Work out the finished part from the listing and answer in its coordinate system (mm). A direction names the side the tool comes from. Coordinates: 2 decimals unless noted, no trailing zeros. Write each loop counter-clockwise with the first axis right and the second up, starting at its lowest first coordinate (ties: lowest second). Pieces come first, ordered by that corner, then holes. Notation, with made-up numbers: (70, -26) - (105, -26) arc R18 ccw to (105, -14) - close; hole circle Ø1 at (-40, 61). An arc over 180 degrees is marked (long way). Use a Markdown table: item, result. Add a question column.
(1) For a pull along X with two mould halves and no side action, classify faces 1 (the face through (0.616, 2.014, 1.088)), 2 (the face through (-1.5, 3, 0)), 3 (the face through (-1.5, -7.4, -0.07)) as released by +X, released by -X, zero draft, split by the parting line, or undercut.
(2) The part is cut by section A-A, the plane z = 0. Give the vertices of the cut face in (x, y).
(3) Given pin 1 Ø3 at (x, y) = (-0.5, -13) entering from +Z; pin 2 Ø0.8 at (x, z) = (0, 0) entering from +Y, each flat-ended and moving along its own axis, determine where each tip first touches the part or whether it passes through.
(4) Find the intervals of material crossed by line 1 (Y direction, x = -1.05, z = 0.8); line 2 (Y direction, x = 0.6, z = 1.85); line 3 (Z direction, x = 0, y = -3.25), in increasing order. Write a range as from..to.
(5) The part is cut by section B-B, the plane y = -12.5. Give the vertices of the cut face in (x, z), then the cut area to 3 significant figures.
(6) A tool of negligible diameter and unlimited length cuts with its end or side. For faces 4 (the face through (0, -15, 0)), 5 (the face through (-2, 0, 0)), 6 (the face through (0, 1, 0)), from which of +Z, -Z, +X, -X, +Y, -Y can it reach the whole face along a straight path? Write none if from no direction.
Autodesk Inventor part; units mm, degrees
ref_plane "YZ Plane" through (0, 0, 0) normal (1, 0, 0) x (0, 1, 0)
ref_plane "XZ Plane" through (0, 0, 0) normal (0, 1, 0) x (-1, 0, 0)
ref_plane "XY Plane" through (0, 0, 0) normal (0, 0, 1) x (1, 0, 0)
sketch "スケッチ1" plane through (0, 0, 0) normal (0, 1, 0) x (-1, 0, 0)
  circle A0 centre (0, 0) radius 2.75
  dimension "d0" = 5.5
extrude "押し出し1" add sketch "スケッチ1" along normal blind 3
sketch "スケッチ2" plane through (0, 0, 0) normal (0, -1, 0) x (1, 0, 0)
  circle A0 centre (0, 0) radius 1.5
  dimension "d3" = 3
extrude "押し出し2" add sketch "スケッチ2" along normal blind 15
fillet "フィレット1" radius 0.5 1 edges at (2.75, 3, 0)
fillet "フィレット1" radius 0.2 1 edges at (2.75, 0, 0)
sketch "スケッチ3" plane through (0, 3, 0) normal (0, 1, 0) x (1, 0, 0)
  line L0 (0, 1.4434) -> (-1.25, 0.7217)
  line L1 (-1.25, 0.7217) -> (-1.25, -0.7217)
  line L2 (-1.25, -0.7217) -> (0, -1.4434)
  line L3 (0, -1.4434) -> (1.25, -0.7217)
  line L4 (1.25, -0.7217) -> (1.25, 0.7217)
  line L5 (1.25, 0.7217) -> (0, 1.4434)
  line L6 (0, 1.4434) -> (0, -1.4434) construction
  circle A0 centre (0, 0) radius 1.4434 construction
  dimension "d12" = 2.5
extrude "押し出し3" cut sketch "スケッチ3" against normal blind 2
thread "ねじ1"
properties part number "M3-CapScrew"
Model answer:
| question | item | result |
|---|---|---|
| 1 | face 1 | undercut |
| 1 | face 2 | zero draft |
| 1 | face 3 | split by the parting line |
| 2 | outline | (-2.75, 0.2) arc R0.2 ccw to (-2.55, 0) - (-1.5, 0) - (-1.5, -15) - (1.5, -15) - (1.5, 0) - (2.55, 0) arc R0.2 ccw to (2.75, 0.2) - (2.75, 2.5) arc R0.5 ccw to (2.25, 3) - (1.25, 3) - (1.25, 1) - (-1.25, 1) - (-1.25, 3) - (-2.25, 3) arc R0.5 ccw to (-2.75, 2.5) - close |
| 3 | pin 1 | z = 1.5 |
| 3 | pin 2 | y = 1 |
| 4 | line 1 | -15..1 |
| 4 | line 2 | 0..3 |
| 4 | line 3 | -1.5..1.5 |
| 5 | outline | circle Ø3 at (0, 0) |
| 5 | area | 7.07 mm^2 |
| 6 | face 4 | +Z, -Z, +X, -X, -Y |
| 6 | face 5 | -Y |
| 6 | face 6 | +Y |
